Check sheet for the modelled part. Datum: model origin and axes. Units: mm. Round coordinates to 2 decimals unless told otherwise and drop trailing zeros. Loops run counter-clockwise (first coordinate to the right, second up) from the corner with the lowest first, then second, coordinate; pieces in that order, holes last. Notation, with made-up numbers: (20, 22) - (37, 22) arc R19 ccw to (37, 41) - close; hole circle Ø4 at (41.25, 44.5). An arc over 180 degrees is marked (long way). Put each result on its own line as item: value.
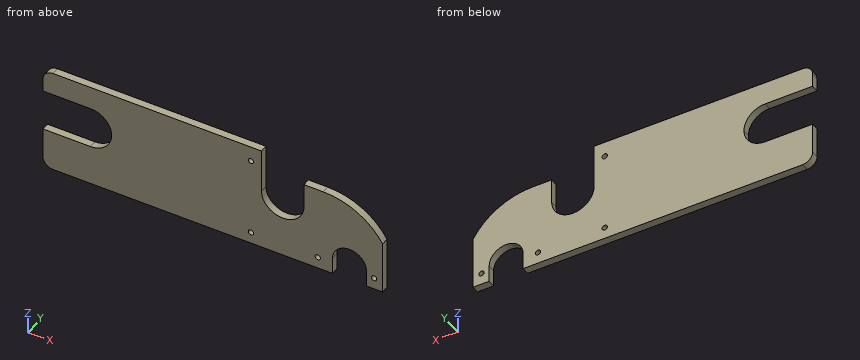
```python
from build123d import *

# Parameters (mm, degrees)
BOSS_EXTRUDE2_DEPTH     = 9.525
CUT_EXTRUDE2_DEPTH      = 453.969139401
F_1_4_CLEARANCE_HOLE1_D = 6.7564


with BuildPart() as part:
    # Sketch1 → Boss-Extrude2 (new body)
    with BuildSketch(Plane(origin=(0, 0, 0), x_dir=(1, 0, 0), z_dir=(0, 1, 0))):
        with BuildLine():
            Line((25.4, 0), (277.8125, 0))
            Line((277.8125, 0), (277.8125, 57.15))
            ThreePointArc((277.8125, 57.15), (304.8, 84.1375), (331.78749993, 57.15))
            Line((331.78749993, 57.15), (331.78749993, 0))
            Line((331.78749993, 0), (357.18749993, 0))
            ThreePointArc((357.18749993, 0), (407.751306336, 19.640432558), (431.8, 68.2625))
            Line((431.8, 68.2625), (431.8, 136.525))
            Line((431.8, 136.525), (411.226, 136.525))
            Line((411.226, 136.525), (411.226, 114.935))
            ThreePointArc((411.226, 114.935), (389.636, 93.345), (368.046, 114.935))
            Line((368.046, 114.935), (368.046, 136.525))
            Line((368.046, 136.525), (23.8125, 136.525))
            Line((23.8125, 136.525), (12.7, 136.525))
            ThreePointArc((12.7, 136.525), (3.719743879, 132.805256121), (0, 123.825))
            Line((0, 123.825), (0, 96.8375))
            Line((0, 96.8375), (0, 84.1375))
            Line((0, 84.1375), (22.225, 84.1375))
            Line((22.225, 84.1375), (60.325, 84.1375))
            ThreePointArc((60.325, 84.1375), (79.408044257, 76.233044257), (87.3125, 57.15))
            ThreePointArc((87.3125, 57.15), (79.408044257, 38.066955743), (60.325, 30.1625))
            Line((60.325, 30.1625), (22.225, 30.1625))
            Line((22.225, 30.1625), (0, 30.1625))
            Line((0, 30.1625), (0, 17.4625))
            Line((0, 17.4625), (0, 12.7))
            ThreePointArc((0, 12.7), (3.719743879, 3.719743879), (12.7, 0))
            Line((12.7, 0), (25.4, 0))
        make_face()
    extrude(amount=BOSS_EXTRUDE2_DEPTH)

    # Sketch2 → Cut-Extrude2 (cut, through all)
    with BuildSketch(Plane(origin=(0, 9.525, 0), x_dir=(1, 0, 0), z_dir=(0, 1, 0))):
        with BuildLine():
            Line((331.78749993, 0), (331.78749993, 25.4))
            Line((331.78749993, 25.4), (356.39375, 25.4))
            ThreePointArc((356.39375, 25.4), (399.762219091, 36.86444095), (431.8, 68.2625))
            ThreePointArc((431.8, 68.2625), (407.751306336, 19.640432558), (357.18749993, 0))
            Line((357.18749993, 0), (331.78749993, 0))
        make_face()
    extrude(amount=-CUT_EXTRUDE2_DEPTH, mode=Mode.SUBTRACT)

    # 1/4 Clearance Hole1 (through all)
    with Locations(Plane(origin=(0, 9.525, 0), x_dir=(1, 0, 0), z_dir=(0, 1, 0))):
        with Locations((420.9542, 121.44375), (349.26905, 121.44375), (264.318750035, 121.44375), (264.318750035, 19.84375)):
            Hole(F_1_4_CLEARANCE_HOLE1_D / 2)


solid = part.part
```
Item 1: Section check C-C on z = -77. Enter the section's corners in (x, y) (3 decimals), then the cut area to 3 significant figures.
Filled sheet:
outline: (78.609, 0) - (286.516, 0) - (286.516, 9.525) - (78.609, 9.525) - close; (323.084, 0) - (431.8, 0) - (431.8, 9.525) - (323.084, 9.525) - close
area: 3,020 mm²
Item 2: Section check D-D on x = 304.8. Enter the section's corners in (y, z) (1 decimal), then the cut area to 3 significant figures.
Filled sheet:
outline: (0, -136.5) - (9.5, -136.5) - (9.5, -84.1) - (0, -84.1) - close
area: 499 mm²
Item 3: Section check A-A on z = -49. Enter the section's corners in (x, y) (1 decimal).
Filled sheet:
outline: (86.1, 0) - (277.8, 0) - (277.8, 9.5) - (86.1, 9.5) - close; (331.8, 0) - (416.3, 0) - (416.3, 9.5) - (331.8, 9.5) - close
Item 4: Section check B-B on y = 2. Count the separate pieces of the cut face and the enclosed holes in it, then the cut area to 3 significant figures.
Filled sheet:
separate pieces: 1
enclosed holes: 4
area: 45,000 mm²
Item 5: Thickness scan on line 1 (Z direction, x = 40.5, y = 3) (1 decimal); line 2 (X direction, y = 1, z = -24); line 3 (X direction, y = 2.5, z = -68.5). Record the ranges inside material, lowest first. Write a range as from..to.
Filled sheet:
line 1: -136.5..-84.1, -30.2..0
line 2: 0..277.81
line 3: 84.81..280.32, 329.28..431.8
Item 6: Go/stop test with flat-tipped pins: pin 1 (2 mm diameter, centred on y = 4, z = -36, fed in from -X); pin 2 (3 mm diameter, centred on y = 4.5, z = -36, fed in from -X). Record where each tip stops, or that it passes through.
Filled sheet:
pin 1: x = 75.74
pin 2: x = 75
